The model under review builds one solid part; all positions refer to its coordinate system, in mm. Face numbers are marked on the shaded views. A direction names the side the tool comes from. Give positions to 0.01 mm unless a question says otherwise; leave off trailing zeros. Loops run counter-clockwise (first coordinate to the right, second up) from the corner with the lowest first, then second, coordinate; pieces in that order, holes last. Notation, with made-up numbers: (45.25, 22) - (62.25, 22) arc R11 cw to (62.25, 43) - close; hole circle Ø6 at (10.25, 46.25). An arc over 180 degrees is marked (long way). Answer as a JSON object with one key per item and string values.
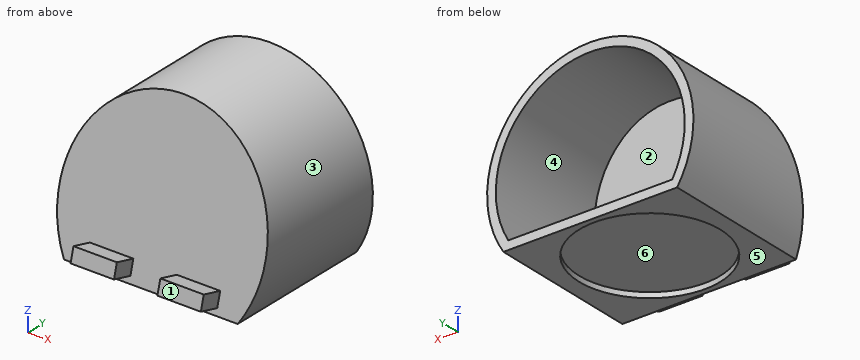
from build123d import *

# Parameters (mm, degrees)
F1_DEPTH = 88.9
F4_DEPTH = 212.726
F5_T     = -5.08
F6_W     = 25.4
F6_H     = 8.382
F7_DEPTH = 12.7
F9_DEPTH = 3.175


with BuildPart() as f1:
    # F0 (on Front) → F1 (new body)
    with BuildSketch(Plane.XZ):
        with BuildLine():
            Line((-50.8, -32.5340686819), (50.8, -32.5340686819))
            ThreePointArc((50.8, -32.5340686819), (0, 60.325), (-50.8, -32.5340686819))
        make_face()
    extrude(amount=-F1_DEPTH)

    # F3 (on offset) → F4 (cut, through all)
    with BuildSketch(Plane.YZ.offset(152.4)):
        Polygon((24.8815124632, 60.325), (0, 60.325), (0, -32.5340686819), align=None)
    extrude(amount=-F4_DEPTH, mode=Mode.SUBTRACT)

    # F5
    f5_openings = [f1.faces().sort_by_distance(p)[0] for p in [
        (0, 88.9, 9.256329),
    ]]
    offset(amount=F5_T, openings=f5_openings)

    # F6 (on face) → F7 (join)
    with BuildSketch(Plane(origin=(0, 8.1335171705, -2.1793693575), x_dir=(1, 0, 0), z_dir=(0, -0.9659258263, 0.2588190451))):
        with Locations((-25.4, -23.4244971741)):
            Rectangle(F6_W, F6_H)
        with Locations((25.4, -23.4244971741)):
            Rectangle(F6_W, F6_H)
    extrude(amount=F7_DEPTH)

    # F8 (on face) → F9 (cut)
    with BuildSketch(Plane(origin=(0, 0, -32.5340686819), x_dir=(1, 0, 0), z_dir=(0, 0, -1))):
        with BuildLine():
            ThreePointArc((41.275, -44.45), (0, -3.175), (-41.275, -44.45))
            Line((-41.275, -44.45), (41.275, -44.45))
        make_face()
        with BuildLine():
            Line((41.275, -44.45), (-41.275, -44.45))
            ThreePointArc((-41.275, -44.45), (0, -85.725), (41.275, -44.45))
        make_face()
    extrude(amount=-F9_DEPTH, mode=Mode.SUBTRACT)


solid = f1.part
Q1. Consider section C-C, the plane y = -5. State the section outline as (x, z) points.
Results:
{"outline": "(-38.1, -27.25) - (-12.7, -27.25) - (-12.7, -18.57) - (-38.1, -18.57) - close; (12.7, -27.25) - (38.1, -27.25) - (38.1, -18.57) - (12.7, -18.57) - close"}
Q2. For the marked faces 4, 5 and 6, list the 3-axis set-ups (+Z, -Z, +X, -X, +Y, -Y) from which the entire face can be reached by the end or side of a thin tool; tool diameter is ignored.
Results:
{"face 4": "+Y", "face 5": "-Z, +X, -X, +Y, -Y", "face 6": "-Z"}
Q3. Clearance check with flat-ended pins moving along their axes: pin 1 Ø8 at (x, z) = (-47.5, -5.5) entering from -Y; pin 2 Ø6 at (x, z) = (-7, 19) entering from -Y; pin 3 Ø12 at (x, z) = (-23.5, 42.5) entering from +Y. State where each tip first meets the part, or that it passes through.
Results:
{"pin 1": "stops at y = 6.17", "pin 2": "stops at y = 13", "pin 3": "stops at y = 26.97"}
Q4. Consider section B-B, the plane x = 0. State the section outline as (y, z) points (3 decimals).
Results:
{"outline": "(0, -32.534) - (3.175, -32.534) - (3.175, -29.359) - (85.725, -29.359) - (85.725, -32.534) - (88.9, -32.534) - (88.9, -27.454) - (6.62, -27.454) - (28.78, 55.245) - (88.9, 55.245) - (88.9, 60.325) - (24.882, 60.325) - close"}
Q5. Consider section D-D, the plane z = 0. State the section outline as (x, y) points (3 decimals), plus the area to 3 significant figures.
Results:
{"outline": "(-60.325, 8.717) - (60.325, 8.717) - (60.325, 88.9) - (55.245, 88.9) - (55.245, 13.977) - (-55.245, 13.977) - (-55.245, 88.9) - (-60.325, 88.9) - close", "area": "1,400 mm^2"}
Q6. Consider section A-A, the plane y = 44.45. State the section outline as (x, z) points (3 decimals), plus the area to 3 significant figures.
Results:
{"outline": "(-50.8, -32.534) - (-41.275, -32.534) - (-41.275, -29.359) - (41.275, -29.359) - (41.275, -32.534) - (50.8, -32.534) arc R60.325 ccw (long way) to start; hole (-47.94, -27.454) - (47.94, -27.454) arc R55.245 ccw (long way) to start", "area": "1,480 mm^2"}
Q7. To check wall thickness, follow probe 1 along X at (y, z) = (35, 0) (3 decimals); probe 2 along Z at (x, y) = (0, 58) (3 decimals); probe 3 along X at (y, z) = (58, 45.5). State the ranges of each line that lie inside material, in increasing order. Write a range as [from, to].
Results:
{"probe 1": "x = [-60.325, -55.245], [55.245, 60.325]", "probe 2": "z = [-29.359, -27.454], [55.245, 60.325]", "probe 3": "x = [-39.61, -31.33], [31.33, 39.61]"}
Q8. The part is to be moulded in two halves that separate along X. For the marked faces 1, 2 and 3, say which applies: +X half, -X half, draft (parallel to the pull), parting line (faces both ways), or undercut.
Results:
{"face 1": "draft", "face 2": "undercut", "face 3": "parting line"}
